from build123d import *

# Parameters (mm, degrees)
SKETCH_1_R          = 6.5
SKETCH_1_R_2        = 2.55
SKETCH_1_W          = 3
SKETCH_1_H          = 20
EXTRUDE_1_DEPTH     = 3
FILLET_1_R          = 1
CHAMFER_1_SIZE      = 1
SKETCH_2_R          = 1.1
CUT_EXTRUDE_1_DEPTH = 68.922750239
FILLET_2_R          = 1


with BuildPart() as part:
    # 草图1 → 凸台-拉伸1 (new body)
    # profile 1 of 4: a face of its own
    with BuildSketch(Plane(origin=(0, 0, 0), x_dir=(1, 0, 0), z_dir=(0, 1, 0))):
        with BuildLine():
            ThreePointArc((6.5, 60), (0, 53.5), (-6.5, 60))
            Line((-6.5, 60), (-6.5, 10))
            Line((-6.5, 10), (-6.5, -10))
            Line((-6.5, -10), (-6.5, -60))
            ThreePointArc((-6.5, -60), (0, -53.5), (6.5, -60))
            Line((6.5, -60), (6.5, -50))
            Line((6.5, -50), (8.5, -50))
            Line((8.5, -50), (8.5, -46))
            ThreePointArc((8.5, -46), (7.5, -45), (8.5, -44))
            Line((8.5, -44), (13.5, -44))
            Line((13.5, -44), (13.5, -34))
            Line((13.5, -34), (8.5, -34))
            ThreePointArc((8.5, -34), (7.5, -33), (8.5, -32))
            Line((8.5, -32), (8.5, -28))
            ThreePointArc((8.5, -28), (7.5, -27), (8.5, -26))
            Line((8.5, -26), (13.5, -26))
            Line((13.5, -26), (13.5, -16))
            Line((13.5, -16), (8.5, -16))
            ThreePointArc((8.5, -16), (7.5, -15), (8.5, -14))
            Line((8.5, -14), (8.5, -10))
            Line((8.5, -10), (-0.5, -10))
            Line((-0.5, -10), (-0.5, 10))
            Line((-0.5, 10), (8.5, 10))
            Line((8.5, 10), (8.5, 14))
            ThreePointArc((8.5, 14), (7.5, 15), (8.5, 16))
            Line((8.5, 16), (13.5, 16))
            Line((13.5, 16), (13.5, 26))
            Line((13.5, 26), (8.5, 26))
            ThreePointArc((8.5, 26), (7.5, 27), (8.5, 28))
            Line((8.5, 28), (8.5, 32))
            ThreePointArc((8.5, 32), (7.5, 33), (8.5, 34))
            Line((8.5, 34), (13.5, 34))
            Line((13.5, 34), (13.5, 44))
            Line((13.5, 44), (8.5, 44))
            ThreePointArc((8.5, 44), (7.5, 45), (8.5, 46))
            Line((8.5, 46), (8.5, 50))
            Line((8.5, 50), (6.5, 50))
            Line((6.5, 50), (6.5, 60))
        make_face()
    # profile 2 of 4: a face of its own
    with BuildSketch(Plane(origin=(0, 0, 0), x_dir=(1, 0, 0), z_dir=(0, 1, 0))):
        with Locations((0, -60)):
            Circle(SKETCH_1_R)
        with Locations(Location((0, -60, 0), (0, 0, 270))):
            Circle(SKETCH_1_R_2, mode=Mode.SUBTRACT)
    # profile 3 of 4: a face of its own
    with BuildSketch(Plane(origin=(0, 0, 0), x_dir=(1, 0, 0), z_dir=(0, 1, 0))):
        with Locations((0, 60)):
            Circle(SKETCH_1_R)
        with Locations(Location((0, 60, 0), (0, 0, 270))):
            Circle(SKETCH_1_R_2, mode=Mode.SUBTRACT)
    # profile 4 of 4: a face of its own
    with BuildSketch(Plane(origin=(0, 0, 0), x_dir=(1, 0, 0), z_dir=(0, 1, 0))):
        with Locations((-8, 0)):
            Rectangle(SKETCH_1_W, SKETCH_1_H)
    extrude(amount=EXTRUDE_1_DEPTH)

    # 圆角1
    fillet_1_edges = [part.edges().sort_by_distance(p)[0] for p in [
        (6.5, 1.5, 50),
        (-6.5, 1.5, 10),
        (-9.5, 1.5, 10),
        (-9.5, 1.5, -10),
        (-6.5, 1.5, -10),
        (6.5, 1.5, -50),
        (-0.5, 1.5, -10),
        (-0.5, 1.5, 10),
    ]]
    fillet(fillet_1_edges, radius=FILLET_1_R)

    # 倒角1
    chamfer_1_edges = [part.edges().sort_by_distance(p)[0] for p in [
        (13.5, 1.5, 16),
        (13.5, 1.5, 26),
        (13.5, 1.5, 34),
        (13.5, 1.5, 44),
        (13.5, 1.5, -44),
        (13.5, 1.5, -34),
        (13.5, 1.5, -26),
        (13.5, 1.5, -16),
    ]]
    chamfer(chamfer_1_edges, length=CHAMFER_1_SIZE)

    # 草图2 → 切除-拉伸1 (cut, through all)
    with BuildSketch(Plane(origin=(0, 3, 0), x_dir=(1, 0, 0), z_dir=(0, 1, 0))):
        with Locations((6.75, 6)):
            Circle(SKETCH_2_R)
        with Locations((-1.25, 6)):
            Circle(SKETCH_2_R)
        with Locations((6.75, -6)):
            Circle(SKETCH_2_R)
        with Locations((-1.25, -6)):
            Circle(SKETCH_2_R)
    extrude(amount=-CUT_EXTRUDE_1_DEPTH, mode=Mode.SUBTRACT)

    # 圆角2
    fillet_2_edges = [part.edges().sort_by_distance(p)[0] for p in [
        (-0.5, 1.5, -6.804673847),
        (-0.5, 1.5, -5.195326153),
        (-0.5, 1.5, 5.195326153),
        (-0.5, 1.5, 6.804673847),
    ]]
    fillet(fillet_2_edges, radius=FILLET_2_R)


solid = part.part
Geometry: final body of the model. Coordinates: model frame, mm. A direction names the side the tool comes from. Coordinates: 2 decimals unless noted, no trailing zeros. Order: outer loops, then holes, each group sorted by start corner. A loop starts at its lowest first (then second) coordinate and runs counter-clockwise, first axis right, second up.
(1) Section query A-A (x = 4.25). Return the cut outline in (y, z).
(2) Section query B-B (y = 2.25). State how many separate pieces and enclosed holes the cut face has, plus the area to 3 significant figures.
(3) Section query C-C (z = -41). Return the cut outline in (x, y).
(4) Material intervals for probe 1 along Z at (x, y) = (9.75, 0.3); probe 2 along X at (y, z) = (1.95, -60); probe 3 along X at (y, z) = (1.1, 53.5), sorted ascending.
(5) Section query D-D (z = 2.5). Return the cut outline in (x, y), plus the area to 3 significant figures.
(6) Draft query along X for faces 4 (the face through (13.5, 1, -21)), 5 (the face through (0.112, 1.479, -62.548)), 6 (the face through (5, 1, 10)). Return one class per face: pulls with the +X half, pulls with the -X half, needs draft (parallel to the pull), parting line crosses it, or undercut.
(7) Access query for faces 1 (the face through (13.5, 1, -39)), 2 (the face through (8.5, 1, 48)), 3 (the face through (10, 1, 26)). Directions: +Z, -Z, +X, -X, +Y, -Y. A direction counts if a zero-diameter tool reaches every point of the face in a straight line with its end or side. Return the directions, or none.
(8) First-contact query: pin 1 (1.5 mm diameter, centred on x = 5, y = 1, fed in from -Z); pin 2 (1.1 mm diameter, centred on x = -8, y = 1, fed in from -Z); pin 3 (0.5 mm diameter, centred on x = -8, y = 1, fed in from +Z). Flat tips, straight axial feed; report the tip coordinate or a pass-through.
Solution:
1. outline: (0, -64.92) - (3, -64.92) - (3, -10) - (0, -10) - close; (0, 10) - (3, 10) - (3, 64.92) - (0, 64.92) - close
2. separate pieces: 1
2. enclosed holes: 2
2. area: 1,910 mm2
3. outline: (-6.5, 0) - (13.5, 0) - (13.5, 3) - (-6.5, 3) - close
4. probe 1: z = -44 to -34, -26 to -16, 16 to 26, 34 to 44
4. probe 2: x = -6.5 to -2.55, 2.55 to 6.5
4. probe 3: x = -6.5 to 6.5
5. outline: (-9.5, 0) - (-0.5, 0) - (-0.5, 3) - (-9.5, 3) - close
5. area: 27.0 mm2
6. face 4: pulls with the +X half
6. face 5: undercut
6. face 6: needs draft
7. face 1: +Z, -Z, +X, +Y, -Y
7. face 2: +Z, +X, +Y, -Y
7. face 3: +X, +Y, -Y
8. pin 1: stops at z = -64.92
8. pin 2: stops at z = -10
8. pin 3: stops at z = 10
